from build123d import *

# Parameters (mm, degrees)
F1_DEPTH = 0.5


with BuildPart() as f1:
    # F0 (on Front) → F1 (new body, symmetric)
    with BuildSketch(Plane.XZ):
        with BuildLine():
            Line((-125, 345), (-233.5, 345))
            ThreePointArc((-233.5, 345), (-237.035534, 343.535534), (-238.5, 340))
            Line((-238.5, 340), (-238.5, 264))
            Line((-238.5, 264), (-241.37868, 261.12132))
            ThreePointArc((-241.37868, 261.12132), (-242.257359, 259), (-241.37868, 256.87868))
            Line((-241.37868, 256.87868), (-238.5, 254))
            Line((-238.5, 254), (-238.5, 178))
            Line((-238.5, 178), (-241.37868, 175.12132))
            ThreePointArc((-241.37868, 175.12132), (-242.257359, 173), (-241.37868, 170.87868))
            Line((-241.37868, 170.87868), (-238.5, 168))
            Line((-238.5, 168), (-238.5, 92))
            Line((-238.5, 92), (-241.37868, 89.12132))
            ThreePointArc((-241.37868, 89.12132), (-242.257359, 87), (-241.37868, 84.87868))
            Line((-241.37868, 84.87868), (-238.5, 82))
            Line((-238.5, 82), (-238.5, 5))
            ThreePointArc((-238.5, 5), (-237.035534, 1.464466), (-233.5, 0))
            Line((-233.5, 0), (233.5, 0))
            ThreePointArc((233.5, 0), (237.035534, 1.464466), (238.5, 5))
            Line((238.5, 5), (238.5, 82))
            Line((238.5, 82), (241.37868, 84.87868))
            ThreePointArc((241.37868, 84.87868), (242.257359, 87), (241.37868, 89.12132))
            Line((241.37868, 89.12132), (238.5, 92))
            Line((238.5, 92), (238.5, 168))
            Line((238.5, 168), (241.37868, 170.87868))
            ThreePointArc((241.37868, 170.87868), (242.257359, 173), (241.37868, 175.12132))
            Line((241.37868, 175.12132), (238.5, 178))
            Line((238.5, 178), (238.5, 254))
            Line((238.5, 254), (241.37868, 256.87868))
            ThreePointArc((241.37868, 256.87868), (242.257359, 259), (241.37868, 261.12132))
            Line((241.37868, 261.12132), (238.5, 264))
            Line((238.5, 264), (238.5, 340))
            ThreePointArc((238.5, 340), (237.035534, 343.535534), (233.5, 345))
            Line((233.5, 345), (125, 345))
            Line((125, 345), (122.12132, 347.87868))
            ThreePointArc((122.12132, 347.87868), (120, 348.757359), (117.87868, 347.87868))
            Line((117.87868, 347.87868), (115, 345))
            Line((115, 345), (5, 345))
            Line((5, 345), (2.12132, 347.87868))
            ThreePointArc((2.12132, 347.87868), (0, 348.757359), (-2.12132, 347.87868))
            Line((-2.12132, 347.87868), (-5, 345))
            Line((-5, 345), (-115, 345))
            Line((-115, 345), (-117.87868, 347.87868))
            ThreePointArc((-117.87868, 347.87868), (-120, 348.757359), (-122.12132, 347.87868))
            Line((-122.12132, 347.87868), (-125, 345))
        make_face()
    extrude(amount=F1_DEPTH, both=True)


solid = f1.part
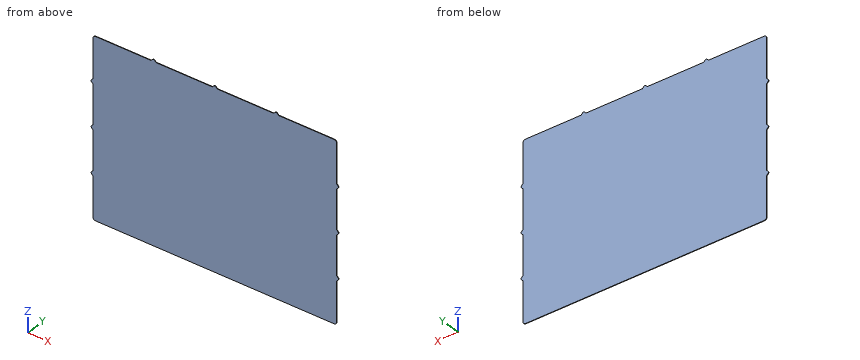
Design review of the part built by this model. Coordinates are the model's own, in mm. Coordinates: 2 decimals unless noted, no trailing zeros. Write each loop counter-clockwise with the first axis right and the second up, starting at its lowest first coordinate (ties: lowest second). Pieces come first, ordered by that corner, then holes. Notation, with made-up numbers: (-3, 52.5) - (27, 52.5) arc R20 cw to (27, 59.5) - close; hole circle Ø8 at (88.5, 23). An arc over 180 degrees is marked (long way). Use one line per item in the form item = value.
Q1. Insertion check: pin 1 Ø0.5 at (x, y) = (53, 0) entering from +Z. The pin has a flat end and moves straight along its axis. Give the tip position at first contact, or say it passes through.
Taken from the geometry:
pin_1 = 345
Q2. Consider section A-A (z = 319.5). Write out the cut boundary in (x, y), plus the area to 3 significant figures.
Taken from the geometry:
outline = (-238.5, -0.5) - (238.5, -0.5) - (238.5, 0.5) - (-238.5, 0.5) - close
area = 477 mm^2
Q3. For probe 1 along Z at (x, y) = (-55, 0.1); probe 2 along X at (y, z) = (0.3, 324.5), list the stretches that pass through material, from the lowest coordinate up.
Taken from the geometry:
probe_1 = 0 to 345
probe_2 = -238.5 to 238.5
